```python
from build123d import *

# Parameters (mm, degrees)
F0_R     = 12.5
F1_DEPTH = 15
F2_R     = 10
F3_R     = 2
F4_W     = 10
F4_H     = 6
F5_DEPTH = 107.001


with BuildPart() as f1:
    # F0 (on Top) → F1 (new body)
    with BuildSketch(Plane.XY):
        with BuildLine():
            ThreePointArc((21.864888, -5.308172), (22.340658, -2.673016), (22.5, 0))
            ThreePointArc((22.5, 0), (21.774068, 5.669212), (19.643114, 10.972606))
            ThreePointArc((19.643114, 10.972606), (13.968986, 17.638521), (6.180399, 21.634525))
            ThreePointArc((6.180399, 21.634525), (3.120352, 22.282581), (0, 22.5))
            ThreePointArc((0, 22.5), (-3.120352, 22.282581), (-6.180399, 21.634525))
            ThreePointArc((-6.180399, 21.634525), (-13.968986, 17.638521), (-19.643114, 10.972606))
            ThreePointArc((-19.643114, 10.972606), (-22.293373, 3.042289), (-21.864888, -5.308172))
            ThreePointArc((-21.864888, -5.308172), (0, -22.5), (21.864888, -5.308172))
        make_face()
        Circle(F0_R, mode=Mode.SUBTRACT)
        with BuildLine():
            ThreePointArc((19.643114, 10.972606), (21.774068, 5.669212), (22.5, 0))
            ThreePointArc((22.5, 0), (22.340658, -2.673016), (21.864888, -5.308172))
            Line((21.864888, -5.308172), (53.5, 125))
            Line((53.5, 125), (53.5, 160))
            Line((53.5, 160), (45.5, 160))
            Line((45.5, 160), (45.5, 125))
            Line((45.5, 125), (0, 22.5))
            ThreePointArc((0, 22.5), (3.120352, 22.282581), (6.180399, 21.634525))
            Line((6.180399, 21.634525), (41.605751, 101.438889))
            Line((41.605751, 101.438889), (19.643114, 10.972606))
        make_face()
        with BuildLine():
            Line((-53.5, 125), (-21.864888, -5.308172))
            ThreePointArc((-21.864888, -5.308172), (-22.293373, 3.042289), (-19.643114, 10.972606))
            Line((-19.643114, 10.972606), (-41.605751, 101.438889))
            Line((-41.605751, 101.438889), (-6.180399, 21.634525))
            ThreePointArc((-6.180399, 21.634525), (-3.120352, 22.282581), (0, 22.5))
            Line((0, 22.5), (-45.5, 125))
            Line((-45.5, 125), (-45.5, 160))
            Line((-45.5, 160), (-53.5, 160))
            Line((-53.5, 160), (-53.5, 125))
        make_face()
    extrude(amount=F1_DEPTH)

    # F2
    f2_edges = [f1.edges().sort_by_distance(p)[0] for p in [
        (-53.5, 125, 7.5),
        (45.5, 125, 7.5),
        (-45.5, 125, 7.5),
        (53.5, 125, 7.5),
    ]]
    fillet(f2_edges, radius=F2_R)

    # F3
    f3_edges = [f1.edges().sort_by_distance(p)[0] for p in [
        (-6.180399, 21.634525, 7.5),
        (-19.643114, 10.972606, 7.5),
        (19.643114, 10.972606, 7.5),
        (6.180399, 21.634525, 7.5),
        (0, 22.5, 7.5),
    ]]
    fillet(f3_edges, radius=F3_R)

    # F4 (on face) → F5 (cut, through all)
    with BuildSketch(Plane(origin=(-53.5, 0, 0), x_dir=(0, -1, 0), z_dir=(-1, 0, 0))):
        with Locations((-150, 7.5)):
            Rectangle(F4_W, F4_H)
    extrude(amount=-F5_DEPTH, mode=Mode.SUBTRACT)


solid = f1.part
```
Part model, mm, in its own coordinate system. A direction names the side the tool comes from. Give positions to 0.01 mm unless a question says otherwise; leave off trailing zeros. Write each loop counter-clockwise with the first axis right and the second up, starting at its lowest first coordinate (ties: lowest second). Pieces come first, ordered by that corner, then holes. Notation, with made-up numbers: M 38.5,59.5 L 83.5,59.5 A17 ccw 83.5,80.5 Z; hole C -35.75,-11.75 d10. An arc over 180 degrees is marked long. Use CSV: the item, a comma, the result in double quotes.
Item 1: Pull direction X, two halves, no side cores. Call faces 1 (the face through (-45.277, 125.017, 7.605)), 2 (the face through (-0.42, -22.496, 7.395)), 3 (the face through (-50, 145, 7)), 4 (the face through (-53.5, 143, 7)): +X half, -X half, draft (parallel to the pull), parting line (faces both ways), or undercut.
Taken from the geometry:
face 1,"undercut"
face 2,"parting line"
face 3,"draft"
face 4,"-X half"
Item 2: Slice it at B-B on y = 136. Write the cut outline in (x, z), plus the area to 3 significant figures.
Taken from the geometry:
outline,"M -53.5,0 L -45.5,0 L -45.5,15 L -53.5,15 Z; M 45.5,0 L 53.5,0 L 53.5,15 L 45.5,15 Z"
area,"240 mm²"
Item 3: Slice it at A-A on x = 0. Write the cut outline in (y, z), plus the area to 3 significant figures.
Taken from the geometry:
outline,"M -22.5,0 L -12.5,0 L -12.5,15 L -22.5,15 Z; M 12.5,0 L 25.43,0 L 25.43,15 L 12.5,15 Z"
area,"344 mm²"
Item 4: Slice it at D-D on y = 45. Write the cut outline in (x, z).
Taken from the geometry:
outline,"M -34.08,0 L -27.9,0 L -27.9,15 L -34.08,15 Z; M -16.55,0 L -9.99,0 L -9.99,15 L -16.55,15 Z; M 9.99,0 L 16.55,0 L 16.55,15 L 9.99,15 Z; M 27.9,0 L 34.08,0 L 34.08,15 L 27.9,15 Z"
Item 5: Which spindle directions (+Z, -Z, +X, -X, +Y, -Y) get a long thin tool onto all of the face, cutting with end or side? Do faces 5 (the face through (-12, 49, 0)), 6 (the face through (-24.58, 63.08, 7.4)), 7 (the face through (-45.5, 143, 7)), 8 (the face through (37.32, 58.36, 7.4)), 9 (the face through (49, 150, 10.5)). Say none if no direction does.
Taken from the geometry:
face 5,"-Z, +X, -X, +Y, -Y"
face 6,"+Z, -Z"
face 7,"+Z, -Z, +Y"
face 8,"+Z, -Z, +X, -Y"
face 9,"+X, -X"
Item 6: Drill centre lines: probe 1 along Y at (x, z) = (0, 4.75); probe 2 along X at (y, z) = (15.5, 2); probe 3 along X at (y, z) = (72, 4.25). Where is each one in solid material? Low to high.
Taken from the geometry:
probe 1,"y = -22.5 to -12.5, 12.5 to 25.43"
probe 2,"x = -26.92 to -20.74, -16.31 to 16.31, 20.74 to 26.92"
probe 3,"x = -40.63 to -34.46, -28.54 to -21.97, 21.97 to 28.54, 34.46 to 40.63"
Item 7: Slice it at C-C on z = 12.25. Write the cut outline in (x, y), plus the area to 3 significant figures.
Taken from the geometry:
outline,"M -53.5,126.2 A10 ccw -53.22,123.84 L -21.86,-5.31 A22.5 ccw 21.86,-5.31 L 53.22,123.84 A10 ccw 53.5,126.2 L 53.5,160 L 45.5,160 L 45.5,127.12 A10 cw 44.64,123.06 L 1.83,26.62 A2 cw -1.83,26.62 L -44.64,123.06 A10 cw -45.5,127.12 L -45.5,160 L -53.5,160 Z; hole M -41.61,101.44 L -20.69,15.3 A2 ccw -17.22,14.48 A22.5 cw -8.17,20.96 A2 ccw -7.07,23.64 Z; hole C 0,0 d25; hole M 7.07,23.64 A2 ccw 8.17,20.96 A22.5 cw 17.22,14.48 A2 ccw 20.69,15.3 L 41.61,101.44 Z"
area,"4,390 mm²"
Item 8: Pin check, flat tips, straight feed: P1, Ø5, axis at y = 63, z = 4.5, coming from the -X side; P2, Ø2, axis at y = 12, z = 6, coming from the -X side; P3, Ø8, axis at y = 56.5, z = 4.5, coming from the +X side. Stop position of each tip, or through.
Taken from the geometry:
P1,"stops at x = -39.06"
P2,"stops at x = -26.31"
P3,"stops at x = 37.84"
